```python
from build123d import *

# Parameters (mm, degrees)
F0_R     = 4.05
F1_DEPTH = 3


with BuildPart() as f1:
    # F0 (on Top) → F1 (new body)
    with BuildSketch(Plane.XY):
        with BuildLine():
            Line((71.412218, -13.5), (91.412218, -13.5))
            ThreePointArc((91.412218, -13.5), (116, 0), (91.412218, 13.5))
            Line((91.412218, 13.5), (71.412218, 13.5))
            Line((71.412218, 13.5), (61.463404, 13.5))
            ThreePointArc((61.463404, 13.5), (51.251366, 16.303655), (43.902431, 23.928571))
            ThreePointArc((43.902431, 23.928571), (35.355339, 35.355339), (23.928571, 43.902431))
            ThreePointArc((23.928571, 43.902431), (16.303655, 51.251366), (13.5, 61.463404))
            Line((13.5, 61.463404), (13.5, 91.412218))
            ThreePointArc((13.5, 91.412218), (0, 116), (-13.5, 91.412218))
            Line((-13.5, 91.412218), (-13.5, 71.412218))
            ThreePointArc((-13.5, 71.412218), (-9.337722, 68.412218), (-13.5, 65.412218))
            Line((-13.5, 65.412218), (-13.5, 61.463404))
            ThreePointArc((-13.5, 61.463404), (-16.303655, 51.251366), (-23.928571, 43.902431))
            ThreePointArc((-23.928571, 43.902431), (-35.355339, 35.355339), (-43.902431, 23.928571))
            ThreePointArc((-43.902431, 23.928571), (-51.251366, 16.303655), (-61.463404, 13.5))
            Line((-61.463404, 13.5), (-65.412218, 13.5))
            ThreePointArc((-65.412218, 13.5), (-68.412218, 9.337722), (-71.412218, 13.5))
            Line((-71.412218, 13.5), (-91.412218, 13.5))
            ThreePointArc((-91.412218, 13.5), (-116, 0), (-91.412218, -13.5))
            Line((-91.412218, -13.5), (-71.412218, -13.5))
            Line((-71.412218, -13.5), (-65.412218, -13.5))
            Line((-65.412218, -13.5), (-61.463404, -13.5))
            ThreePointArc((-61.463404, -13.5), (-51.251366, -16.303655), (-43.902431, -23.928571))
            ThreePointArc((-43.902431, -23.928571), (-35.355339, -35.355339), (-23.928571, -43.902431))
            ThreePointArc((-23.928571, -43.902431), (-16.303655, -51.251366), (-13.5, -61.463404))
            Line((-13.5, -61.463404), (-13.5, -91.412218))
            ThreePointArc((-13.5, -91.412218), (0, -116), (13.5, -91.412218))
            Line((13.5, -91.412218), (13.5, -71.412218))
            ThreePointArc((13.5, -71.412218), (9.337722, -68.412218), (13.5, -65.412218))
            Line((13.5, -65.412218), (13.5, -61.463404))
            ThreePointArc((13.5, -61.463404), (16.303655, -51.251366), (23.928571, -43.902431))
            ThreePointArc((23.928571, -43.902431), (35.355339, -35.355339), (43.902431, -23.928571))
            ThreePointArc((43.902431, -23.928571), (51.251366, -16.303655), (61.463404, -13.5))
            Line((61.463404, -13.5), (65.412218, -13.5))
            ThreePointArc((65.412218, -13.5), (68.412218, -9.337722), (71.412218, -13.5))
        make_face()
        with BuildLine():
            Line((-9.193748, -103.575962), (-7.461697, -102.575962))
            ThreePointArc((-7.461697, -102.575962), (-5.412659, -103.125), (-5.961697, -105.174038))
            Line((-5.961697, -105.174038), (-7.693748, -106.174038))
            ThreePointArc((-7.693748, -106.174038), (-9.742786, -105.625), (-9.193748, -103.575962))
        make_face(mode=Mode.SUBTRACT)
        with BuildLine():
            ThreePointArc((-2.575962, -92.538303), (-3.125, -94.587341), (-5.174038, -94.038303))
            Line((-5.174038, -94.038303), (-6.174038, -92.306252))
            ThreePointArc((-6.174038, -92.306252), (-5.625, -90.257214), (-3.575962, -90.806252))
            Line((-3.575962, -90.806252), (-2.575962, -92.538303))
        make_face(mode=Mode.SUBTRACT)
        with BuildLine():
            Line((-109.193748, -3.575962), (-107.461697, -2.575962))
            ThreePointArc((-107.461697, -2.575962), (-105.412659, -3.125), (-105.961697, -5.174038))
            Line((-105.961697, -5.174038), (-107.693748, -6.174038))
            ThreePointArc((-107.693748, -6.174038), (-109.742786, -5.625), (-109.193748, -3.575962))
        make_face(mode=Mode.SUBTRACT)
        with BuildLine():
            Line((-96.424038, -9.193748), (-97.424038, -7.461697))
            ThreePointArc((-97.424038, -7.461697), (-96.875, -5.412659), (-94.825962, -5.961697))
            Line((-94.825962, -5.961697), (-93.825962, -7.693748))
            ThreePointArc((-93.825962, -7.693748), (-94.375, -9.742786), (-96.424038, -9.193748))
        make_face(mode=Mode.SUBTRACT)
        with BuildLine():
            Line((3.575962, -109.193748), (2.575962, -107.461697))
            ThreePointArc((2.575962, -107.461697), (3.125, -105.412659), (5.174038, -105.961697))
            Line((5.174038, -105.961697), (6.174038, -107.693748))
            ThreePointArc((6.174038, -107.693748), (5.625, -109.742786), (3.575962, -109.193748))
        make_face(mode=Mode.SUBTRACT)
        with Locations((0, -100)):
            Circle(F0_R, mode=Mode.SUBTRACT)
        with BuildLine():
            Line((9.193748, -96.424038), (7.461697, -97.424038))
            ThreePointArc((7.461697, -97.424038), (5.412659, -96.875), (5.961697, -94.825962))
            Line((5.961697, -94.825962), (7.693748, -93.825962))
            ThreePointArc((7.693748, -93.825962), (9.742786, -94.375), (9.193748, -96.424038))
        make_face(mode=Mode.SUBTRACT)
        with BuildLine():
            ThreePointArc((92.538303, -2.575962), (94.587341, -3.125), (94.038303, -5.174038))
            Line((94.038303, -5.174038), (92.306252, -6.174038))
            ThreePointArc((92.306252, -6.174038), (90.257214, -5.625), (90.806252, -3.575962))
            Line((90.806252, -3.575962), (92.538303, -2.575962))
        make_face(mode=Mode.SUBTRACT)
        with BuildLine():
            ThreePointArc((102.575962, -7.461697), (103.125, -5.412659), (105.174038, -5.961697))
            Line((105.174038, -5.961697), (106.174038, -7.693748))
            ThreePointArc((106.174038, -7.693748), (105.625, -9.742786), (103.575962, -9.193748))
            Line((103.575962, -9.193748), (102.575962, -7.461697))
        make_face(mode=Mode.SUBTRACT)
        with BuildLine():
            Line((-103.575962, 9.193748), (-102.575962, 7.461697))
            ThreePointArc((-102.575962, 7.461697), (-103.125, 5.412659), (-105.174038, 5.961697))
            Line((-105.174038, 5.961697), (-106.174038, 7.693748))
            ThreePointArc((-106.174038, 7.693748), (-105.625, 9.742786), (-103.575962, 9.193748))
        make_face(mode=Mode.SUBTRACT)
        with Locations((-100, 0)):
            Circle(F0_R, mode=Mode.SUBTRACT)
        with BuildLine():
            ThreePointArc((-92.538303, 2.575962), (-94.587341, 3.125), (-94.038303, 5.174038))
            Line((-94.038303, 5.174038), (-92.306252, 6.174038))
            ThreePointArc((-92.306252, 6.174038), (-90.257214, 5.625), (-90.806252, 3.575962))
            Line((-90.806252, 3.575962), (-92.538303, 2.575962))
        make_face(mode=Mode.SUBTRACT)
        with BuildLine():
            Line((-9.193748, 96.424038), (-7.461697, 97.424038))
            ThreePointArc((-7.461697, 97.424038), (-5.412659, 96.875), (-5.961697, 94.825962))
            Line((-5.961697, 94.825962), (-7.693748, 93.825962))
            ThreePointArc((-7.693748, 93.825962), (-9.742786, 94.375), (-9.193748, 96.424038))
        make_face(mode=Mode.SUBTRACT)
        with BuildLine():
            Line((-3.575962, 109.193748), (-2.575962, 107.461697))
            ThreePointArc((-2.575962, 107.461697), (-3.125, 105.412659), (-5.174038, 105.961697))
            Line((-5.174038, 105.961697), (-6.174038, 107.693748))
            ThreePointArc((-6.174038, 107.693748), (-5.625, 109.742786), (-3.575962, 109.193748))
        make_face(mode=Mode.SUBTRACT)
        with BuildLine():
            ThreePointArc((27.692199, 16.035651), (-22.627417, -22.627417), (16.035651, 27.692199))
            ThreePointArc((16.035651, 27.692199), (16.666653, 27.566052), (17.243872, 27.850474))
            Line((17.243872, 27.850474), (19.522285, 30.128887))
            Line((19.522285, 30.128887), (30.128887, 19.522285))
            Line((30.128887, 19.522285), (27.850474, 17.243872))
            ThreePointArc((27.850474, 17.243872), (27.566052, 16.666653), (27.692199, 16.035651))
        make_face(mode=Mode.SUBTRACT)
        with Locations((100, 0)):
            Circle(F0_R, mode=Mode.SUBTRACT)
        with BuildLine():
            Line((96.424038, 9.193748), (97.424038, 7.461697))
            ThreePointArc((97.424038, 7.461697), (96.875, 5.412659), (94.825962, 5.961697))
            Line((94.825962, 5.961697), (93.825962, 7.693748))
            ThreePointArc((93.825962, 7.693748), (94.375, 9.742786), (96.424038, 9.193748))
        make_face(mode=Mode.SUBTRACT)
        with BuildLine():
            ThreePointArc((107.461697, 2.575962), (105.412659, 3.125), (105.961697, 5.174038))
            Line((105.961697, 5.174038), (107.693748, 6.174038))
            ThreePointArc((107.693748, 6.174038), (109.742786, 5.625), (109.193748, 3.575962))
            Line((109.193748, 3.575962), (107.461697, 2.575962))
        make_face(mode=Mode.SUBTRACT)
        with BuildLine():
            ThreePointArc((2.575962, 92.538303), (3.125, 94.587341), (5.174038, 94.038303))
            Line((5.174038, 94.038303), (6.174038, 92.306252))
            ThreePointArc((6.174038, 92.306252), (5.625, 90.257214), (3.575962, 90.806252))
            Line((3.575962, 90.806252), (2.575962, 92.538303))
        make_face(mode=Mode.SUBTRACT)
        with Locations((0, 100)):
            Circle(F0_R, mode=Mode.SUBTRACT)
        with BuildLine():
            Line((9.193748, 103.575962), (7.461697, 102.575962))
            ThreePointArc((7.461697, 102.575962), (5.412659, 103.125), (5.961697, 105.174038))
            Line((5.961697, 105.174038), (7.693748, 106.174038))
            ThreePointArc((7.693748, 106.174038), (9.742786, 105.625), (9.193748, 103.575962))
        make_face(mode=Mode.SUBTRACT)
    extrude(amount=F1_DEPTH)


solid = f1.part
```
Can you work these out from the model? Positions are in its coordinate system, mm. A direction names the side the tool comes from. Give positions to 0.01 mm unless a question says otherwise; leave off trailing zeros. Use CSV: the item, a comma, the result in double quotes. Start each with the question number.
1. If we mould it in two halves opening along Y, with no side actions, what happens to faces 4 (the face through (-116, 0, 1)), 5 (the face through (16.23, -51.38, 1.48)), 6 (the face through (51.38, 16.23, 1.48))? For each: released by +Y, released by -Y, zero draft, split by the parting line, or undercut.
2. On a 3-axis mill with a long thin cutter (end or side, diameter ignored), from which of +Z, -Z, +X, -X, +Y, -Y can I reach the whole of each face in a straight line? I mean faces 1 (the face through (-16.381, -51.123, 1.479)), 2 (the face through (51.123, -16.381, 1.479)), 3 (the face through (24.75, 24.9, 1.48)). Say none if no direction works.
3. If I drill on L1, parallel to Y at x = 0, z = 1.7; L2, parallel to Y at x = 2, z = 1.55; L3, parallel to X at y = -12.5, z = 0.9, over which ranges is the centre line in solid material (lowest first)?
4. Imagine slicing it at A-A, the plane z = 0.75. Count the separate pieces of the cut face and the enclosed holes in it, plus the area to 3 significant figures.
5. For P1, Ø13, axis at x = 0, y = -100, coming from the -Z side; P2, Ø1, axis at x = 68.5, z = 1.5, coming from the -Y side; P3, Ø1, axis at x = -80.5, z = 1, coming from the +Y side; P4, Ø0.9, axis at y = 84, z = 2, coming from the -X side, each with a flat end and sliding along its axis, tell me the tip position at first contact or that it passes through.
Response values:
1,face 4,"split by the parting line"
1,face 5,"undercut"
1,face 6,"released by +Y"
2,face 1,"+Z, -Z, -X"
2,face 2,"+Z, -Z, -Y"
2,face 3,"+Z, -Z"
3,L1,"-116 to -104.05, -95.95 to -32, 32 to 95.95, 104.05 to 116"
3,L2,"-115.87 to -103.52, -96.48 to -31.94, 31.94 to 96.48, 103.52 to 115.87"
3,L3,"-109.99 to -29.46, 29.46 to 65.25, 71.57 to 109.99"
4,separate pieces,"1"
4,enclosed holes,"21"
4,area,"11,500 mm^2"
5,P1,"z = 0"
5,P2,"y = -9.39"
5,P3,"y = 13.5"
5,P4,"x = -13.5"
